Autodesk Inventor part; units mm, degrees
ref_plane "YZ Plane" through (0, 0, 0) normal (1, 0, 0) x (0, 1, 0)
ref_plane "XZ Plane" through (0, 0, 0) normal (0, 1, 0) x (-1, 0, 0)
ref_plane "XY Plane" through (0, 0, 0) normal (0, 0, 1) x (1, 0, 0)
sketch "Sketch2" plane through (0, 0, 0) normal (1, 0, 0) x (0, 1, 0)
  line L0 (17, -27.5) -> (-17, -27.5)
  line L1 (-17, -27.5) -> (-17, 27.5)
  line L2 (-17, 27.5) -> (17, 27.5)
  line L3 (17, 27.5) -> (17, -27.5)
  line L4 (17, -27.5) -> (-17, 27.5) construction
  line L5 (-17, -27.5) -> (17, 27.5) construction
  line L6 (9, 27.5) -> (-9, 27.5)
  line L7 (-9, 27.5) -> (-9, -7.5)
  line L8 (-9, -7.5) -> (9, -7.5)
  line L9 (9, -7.5) -> (9, 27.5)
  point P0 (0, 0)
  point P1 (-9, 27.5)
  dimension "d1" = 34
  dimension "d2" = 55
  dimension "d3" = 8
  dimension "d4" = 8
  dimension "d5" = 20
extrude "Extrusion1" add sketch "Sketch2" along normal mid plane 65 contours L0 L1 L2 L7 L8 L9 L3
sketch "Sketch3" plane through (0, 0, 0) normal (0, 1, 0) x (-1, 0, 0)
  line L0 (32.5, 27.5) -> (-32.5, 27.5)
  line L1 (32.5, 27.5) -> (-2.5, 27.5)
  line L2 (-2.5, 27.5) -> (-2.5, -7.5)
  line L3 (-2.5, -7.5) -> (32.5, -7.5)
  line L4 (32.5, -7.5) -> (32.5, 27.5)
  point P0 (0, 0)
  dimension "d8" = 35
  dimension "d9" = 35
extrude "Extrusion2" cut sketch "Sketch3" along normal through all both and the other way through all
sketch "Sketch4" plane through (32.5, 0, 0) normal (1, 0, 0) x (0, 0, -1)
  line L0 (21, -17) -> (14, -17)
  line L1 (14, -17) -> (14, -20)
  line L2 (14, -20) -> (21, -20)
  line L3 (21, -20) -> (21, -17)
  line L4 (27.5, -17) -> (27.5, 17)
  line L5 (-27.5, -17) -> (27.5, -17)
  line L6 (27.5, 17) -> (27.5, -17)
  line L7 (27.5, 0) -> (7.5, 0) construction
  line L8 (7.5, -17) -> (7.5, 17)
  line L9 (21, 17) -> (14, 17)
  line L10 (14, 17) -> (14, 20)
  line L11 (14, 20) -> (21, 20)
  line L12 (21, 20) -> (21, 17)
  point P0 (0, 0)
  dimension "d12" = 7
  dimension "d13" = 3
  dimension "d14" = 6.5
extrude "Extrusion3" add sketch "Sketch4" against normal blind 6
extrude "Extrusion4" add sketch "Sketch4" along normal blind 6 from surface at -65
sketch "Sketch5" plane through (-32.5, -17, -27.5) normal (0, -1, 0) x (1, 0, 0)
  line L0 (65, 0) -> (0, 0)
  line L1 (65, 6.5) -> (65, 0)
  point P0 (32.5, 27.5)
  point P1 (13, 10)
  point P2 (32.5, 10)
  point P3 (52, 10)
  dimension "d19" = 10
  dimension "d20" = 13
  dimension "d21" = 19.5
  dimension "d22" = 19.5
hole "Hole1" at (-19.5, -17, -17.5) at (0, -17, -17.5) at (19.5, -17, -17.5) direction (0, 1, 0) diameter 6.6 end through all counterbore diameter 11 counterbore depth 6.5
sketch "Sketch6" plane through (-32.5, 17, -27.5) normal (0, 1, 0) x (1, 0, 0)
  circle A0 centre (52, -10) radius 3.3
  circle A1 centre (32.5, -10) radius 3.3
  circle A2 centre (13, -10) radius 3.3
  point P0 (32.5, -27.5)
hole "Hole2" at (19.5, 17, -17.5) at (0, 17, -17.5) at (-19.5, 17, -17.5) direction (0, -1, 0) diameter 6.6 end through all counterbore diameter 11 counterbore depth 6.5
sketch "Sketch7" plane through (-32.5, -17, -27.5) normal (0, -1, 0) x (1, 0, 0)
  line L0 (65, 0) -> (0, 0)
  line L1 (65, 55) -> (65, 13.5)
  point P0 (32.5, 27.5)
  point P1 (61, 29)
  dimension "d37" = 29
  dimension "d38" = 4
hole "Hole3" at (28.5, -17, 1.5) direction (0, 1, 0) diameter 3 end through all
sketch "Sketch8" plane through (-32.5, -17, -27.5) normal (0, -1, 0) x (1, 0, 0)
  line L0 (35, 55) -> (65, 55)
  line L1 (65, 55) -> (65, 13.5)
  point P0 (32.5, 27.5)
  point P1 (55, 45)
  dimension "d46" = 10
  dimension "d47" = 10
hole "Hole4" at (22.5, -17, 17.5) direction (0, 1, 0) diameter 8 end through all
sketch "Sketch9" plane through (32.5, -17, 27.5) normal (0, 0, 1) x (1, 0, 0)
  line L0 (-30, 34) -> (0, 34)
  line L1 (-30, 0) -> (0, 0)
  line L2 (0, 8) -> (0, 0)
  point P0 (-32.5, 17)
  point P1 (-10, 4)
  point P2 (-10, 30)
  dimension "d55" = 4
  dimension "d56" = 4
  dimension "d57" = 10
hole "Hole5" at (22.5, -13, 27.5) at (22.5, 13, 27.5) direction (0, 0, -1) diameter 3.242 depth 10 tip angle 118
chamfer "Chamfer1" distance 10 angle 45 2 edges at (2.5, -13, 27.5) (2.5, 13, 27.5)
chamfer "Chamfer2" distance 3 angle 45 2 edges at (32.5, -13, 27.5) (32.5, 13, 27.5)
sketch "Sketch10" plane through (-32.5, 17, -27.5) normal (0, 1, 0) x (1, 0, 0)
  circle A0 centre (53, -29) radius 2.5 construction
  line L0 (0, 0) -> (65, 0)
  line L1 (65, 0) -> (65, -6.5)
  dimension "d71" = 5
  dimension "d72" = 29
  dimension "d74" = 12
hole "Hole6" at (20.5, 17, 1.5) direction (0, -1, 0) diameter 4.134 end through all
properties part number "TL20240701-10200AT-001" material "AL6061"
Geometry check sheet. Reference: the model listing, model coordinates, mm. A direction names the side the tool comes from. Coordinates: 2 decimals unless noted, no trailing zeros. Order: outer loops, then holes, each group sorted by start corner. A loop starts at its lowest first (then second) coordinate and runs counter-clockwise, first axis right, second up. Notation, with made-up numbers: (41.5, 12.25) - (78.5, 12.25) arc R24 cw to (78.5, 38.25) - close; hole circle Ø1 at (49, 32). An arc over 180 degrees is marked (long way). One line per item, written item: value.
(1) Access from +Z, -Z, +X, -X, +Y, -Y to the whole of each face (thin tool, end or side, straight path). Record for faces 1 (the face through (3.3, -13.7, -13.1)), 2 (the face through (30, -19, -21)), 3 (the face through (23.938, -13.748, 24.284)).
Data:
face 1: -Y
face 2: -Z, +X, -X, -Y
face 3: +Z
(2) Sectioned sample at C-C (y = 3). Enter the section's corners in (x, z), and give its area (3 significant figures).
Data:
outline: (-32.5, -27.5) - (32.5, -27.5) - (32.5, -7.5) - (-32.5, -7.5) - close; hole circle Ø6.6 at (-19.5, -17.5); hole circle Ø6.6 at (0, -17.5); hole circle Ø6.6 at (19.5, -17.5)
area: 1,200 mm^2
(3) Release check for a two-part mould opening along Y. For faces 4 (the face through (-17, -10.5, -20)), 5 (the face through (31, -13, 26)), 6 (the face through (17, 9, 10)) record: +Y half, -Y half, draft (parallel to the pull), parting line (faces both ways), or undercut.
Data:
face 4: -Y half
face 5: draft
face 6: undercut
(4) Sectioned sample at A-A (z = 5). Enter the section's corners in (x, y), and give its area (3 significant figures).
Data:
outline: (2.5, -17) - (32.5, -17) - (32.5, -9) - (2.5, -9) - close; (2.5, 9) - (32.5, 9) - (32.5, 17) - (2.5, 17) - close
area: 480 mm^2
(5) Thickness scan on probe 1 along X at (y, z) = (-15.5, -17.5); probe 2 along Y at (x, z) = (22.5, 25); probe 3 along Y at (x, z) = (14, 18). Record the ranges inside material, lowest first. Write a range as from..to.
Data:
probe 1: x = -32.5..-25, -14..-5.5, 5.5..14, 25..32.5
probe 2: y = -17..-14.62, -11.38..-9, 9..11.38, 14.62..17
probe 3: y = -17..-9, 9..17
(6) Depth check by flat-ended pin: pin 1 Ø5.5 at (x, z) = (19.5, -15) entering from +Y; pin 2 Ø1.9 at (x, y) = (22.5, -13) entering from +Z; pin 3 Ø9 at (x, z) = (-20, -18) entering from -Y. Enter the tip coordinate at first touch or a pass-through.
Data:
pin 1: stops at y = 10.5
pin 2: stops at z = 13.61
pin 3: stops at y = -10.5
(7) Sectioned sample at D-D (y = -13). Enter the section's corners in (x, z).
Data:
outline: (-32.5, -27.5) - (32.5, -27.5) - (32.5, 24.5) - (29.5, 27.5) - (24.12, 27.5) - (24.12, 21.16) arc R4 cw (long way) to (20.88, 21.16) - (20.88, 27.5) - (12.5, 27.5) - (2.5, 17.5) - (2.5, -7.5) - (-32.5, -7.5) - close; hole circle Ø11 at (-19.5, -17.5); hole circle Ø11 at (0, -17.5); hole circle Ø11 at (19.5, -17.5); hole circle Ø4.13 at (20.5, 1.5); hole circle Ø3 at (28.5, 1.5)
(8) Sectioned sample at B-B (x = -19.5). Enter the section's corners in (y, z).
Data:
outline: (-17, -27.5) - (17, -27.5) - (17, -23) - (10.5, -23) - (10.5, -20.8) - (-10.5, -20.8) - (-10.5, -23) - (-17, -23) - close; (-17, -12) - (-10.5, -12) - (-10.5, -14.2) - (10.5, -14.2) - (10.5, -12) - (17, -12) - (17, -7.5) - (-17, -7.5) - close
